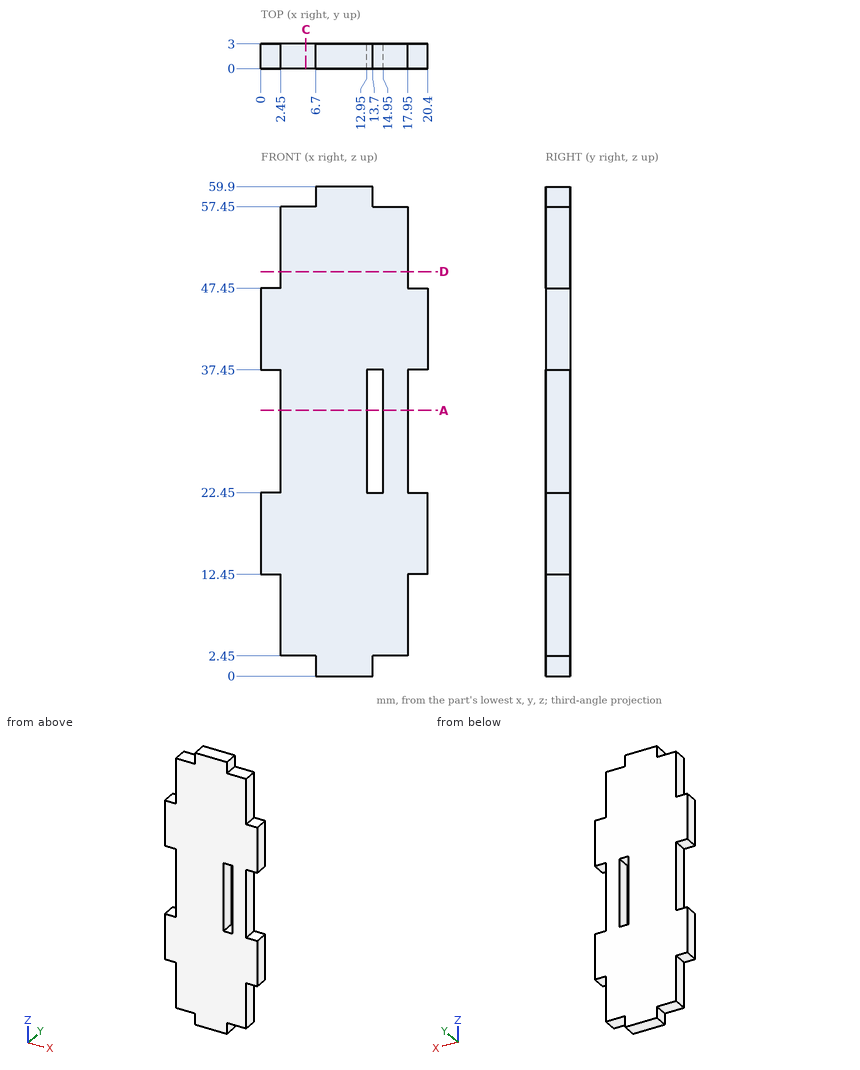
Job drawing, mm, ordinate dimensions from the low corner. One solid piece. Give positions to 0.01 mm unless a question says otherwise; leave off trailing zeros. Loops run counter-clockwise (first coordinate to the right, second up) from the corner with the lowest first, then second, coordinate; pieces in that order, holes last. Notation, with made-up numbers: (87.25, 85.5) -> (96.25, 85.5) arc R28 ccw to (96.25, 113.5) -> close; hole circle Ø1 at (51, -5.5). An arc over 180 degrees is marked (long way). Write each question's results on one line, items separated by ' | '. Start each with the question number.
Q1. Band-saw the part on C-C on x = 5.5. List the corners of the cut face in (y, z), plus the area to 3 significant figures.
Q2. Band-saw the part on D-D on z = 49.5. List the corners of the cut face in (x, y), plus the area to 3 significant figures.
Q3. Band-saw the part on A-A on z = 32.5. List the corners of the cut face in (x, y), plus the area to 3 significant figures.
Q4. Wall check: L1, parallel to X at y = 2, z = 35; L2, parallel to Z at x = 13.25, y = 1.15; L3, parallel to Z at x = 18, y = 2.5. Give the ranges that are in metal, low to high.
Q5. Pin check, flat tips, straight feed: P1, Ø1.5, axis at x = 16.5, y = 1, coming from the +Z side; P2, Ø0.9, axis at x = 15, y = 1, coming from the -Z side; P3, Ø0.9, axis at y = 1.5, z = 28, coming from the -X side; P4, Ø1.5, axis at x = 9.5, z = 20.5, coming from the -Y side. Stop position of each tip, or through.
Results are:
1) outline: (0, 2.45) -> (3, 2.45) -> (3, 57.45) -> (0, 57.45) -> close | area: 165 mm²
2) outline: (2.45, 0) -> (17.95, 0) -> (17.95, 3) -> (2.45, 3) -> close | area: 46.5 mm²
3) outline: (2.45, 0) -> (12.95, 0) -> (12.95, 3) -> (2.45, 3) -> close; (14.95, 0) -> (17.95, 0) -> (17.95, 3) -> (14.95, 3) -> close | area: 40.5 mm²
4) L1: x = 2.45 to 12.95, 14.95 to 17.95 | L2: z = 0 to 22.45, 37.45 to 59.9 | L3: z = 12.45 to 22.45, 37.45 to 47.45
5) P1: stops at z = 57.45 | P2: stops at z = 2.45 | P3: stops at x = 2.45 | P4: stops at y = 0
